Design review of the part built by this model. Coordinates are the model's own, in mm. A direction names the side the tool comes from. Give positions to 0.01 mm unless a question says otherwise; leave off trailing zeros. Write each loop counter-clockwise with the first axis right and the second up, starting at its lowest first coordinate (ties: lowest second). Pieces come first, ordered by that corner, then holes. Notation, with made-up numbers: M 50.5,4 L 70.5,4 A25 cw 70.5,24 Z; hole C 84.5,18.5 d2. An arc over 180 degrees is marked long. Use a Markdown table: item, result. Add a question column.
```python
from build123d import *

# Parameters (mm, degrees)
SKETCH1_W               = 19.05
SKETCH1_H               = 19.05
SKETCH1_W_2             = 15.748
SKETCH1_H_2             = 15.748
BOSS_EXTRUDE1_DEPTH     = 28.575
CUT_EXTRUDE5_DEPTH      = 36.639286609
CUT_EXTRUDE5_DEPTH_BACK = 36.639286609
SKETCH5_R               = 12.7
CUT_EXTRUDE2_DEPTH      = 36.639286609
CUT_EXTRUDE2_DEPTH_BACK = 36.639286609
SKETCH3_R               = 4.064
CUT_EXTRUDE4_DEPTH      = 36.639286609
CUT_EXTRUDE4_DEPTH_BACK = 36.639286609
SKETCH4_W               = 15.748
SKETCH4_H               = 19.05
FILLET2_R               = 6.35


with BuildPart() as part:
    # Sketch1 → Boss-Extrude1 (new body)
    with BuildSketch(Plane.XY):
        Rectangle(SKETCH1_W, SKETCH1_H)
        Rectangle(SKETCH1_W_2, SKETCH1_H_2, mode=Mode.SUBTRACT)
    extrude(amount=BOSS_EXTRUDE1_DEPTH)

    # Sketch5 → Cut-Extrude5 (cut, two sides: drawn at the far end of the back side and taken through both)
    with BuildSketch(Plane(origin=(0, 9.525, 0), x_dir=(1, 0, 0), z_dir=(0, 1, 0)).offset(-CUT_EXTRUDE5_DEPTH_BACK)):
        with Locations((0, 8.400260413)):
            Circle(SKETCH5_R)
    extrude(amount=CUT_EXTRUDE5_DEPTH + CUT_EXTRUDE5_DEPTH_BACK, mode=Mode.SUBTRACT)

    # Sketch3 → Cut-Extrude2 (cut, two sides: drawn at the far end of the back side and taken through both)
    with BuildSketch(Plane(origin=(9.525, 0, 0), x_dir=(0, 0, -1), z_dir=(1, 0, 0)).offset(-CUT_EXTRUDE2_DEPTH_BACK)):
        with Locations(Location((-20.6375, 0, 0), (0, 0, 90))):
            Circle(SKETCH3_R)
    extrude(amount=CUT_EXTRUDE2_DEPTH + CUT_EXTRUDE2_DEPTH_BACK, mode=Mode.SUBTRACT)

    # Sketch4 → Cut-Extrude4 (cut, two sides: drawn at the far end of the back side and taken through both)
    with BuildSketch(Plane.XZ.offset(9.525).offset(-CUT_EXTRUDE4_DEPTH_BACK)):
        with Locations((0, 19.05)):
            Rectangle(SKETCH4_W, SKETCH4_H)
    extrude(amount=CUT_EXTRUDE4_DEPTH + CUT_EXTRUDE4_DEPTH_BACK, mode=Mode.SUBTRACT)

    # Fillet2
    fillet2_edges = [part.edges().sort_by_distance(p)[0] for p in [
        (-8.6995, -9.525, 28.575),
        (8.6995, -9.525, 28.575),
        (-8.6995, 9.525, 28.575),
        (8.6995, 9.525, 28.575),
    ]]
    fillet(fillet2_edges, radius=FILLET2_R)


solid = part.part
```
(1) Wall thickness on L1, parallel to X at y = 0, z = 6 (3 decimals); L2, parallel to Z at x = 8.6, y = 0 (1 decimal): over which ranges is each line inside the solid? List them lowest first.
(2) For pin 1 (1.3 mm diameter, centred on x = 0.5, y = 8.5, fed in from +Z) (3 decimals); pin 2 (5 mm diameter, centred on y = 0, z = 20.64, fed in from +X), all flat-tipped, find the tip position at first contact; note any pin that passes through.
(3) Add section C-C on z = 12.75. Give the boundary of the cut face in (x, y) (3 decimals), then the cut area to 3 significant figures.
(4) The part is to be moulded in two halves that separate along X. For faces 1 (the flat face through (0, -7.874, 6)), 2 (the flat face through (9.525, 0, 14)), 3 (the flat face through (-9.525, 0, 14)), 4 (the cylindrical face through (8.688, 2.185, 24.064)), say which applies: released by +X, released by -X, zero draft, split by the parting line, or undercut.
(5) Add section B-B on y = 0. Give the boundary of the cut face in (x, z) (1 decimal).
(6) Add section A-A on z = 7.25. Give the boundary of the cut face in (x, y) (3 decimals), then the cut area to 3 significant figures.
(7) Machinability: for faces 5 (the flat face through (0, 9, 9.525)), 6 (the cylindrical face through (8.71, -7.62, 26.76)), 7 (the flat face through (-7.874, 0, 15)), 8 (the flat face through (0, 7.874, 6)), which of the approach directions +Z, -Z, +X, -X, +Y, -Y give a long, thin tool a straight path to every point of the face, cutting with its end or side? Answer none if there is none.
(8) Add section D-D on y = 5.25. Give the boundary of the cut face in (x, z) (3 decimals), then the cut area to 3 significant figures.
From the geometry:
| question | item | result |
|---|---|---|
| 1 | L1 | x = -9.525 to -7.874, 7.874 to 9.525 |
| 1 | L2 | z = 0.9 to 16.6, 24.7 to 28.6 |
| 2 | pin 1 | stops at z = 9.525 |
| 2 | pin 2 | passes through |
| 3 | outline | M -9.525,-9.525 L -7.874,-9.525 L -7.874,9.525 L -9.525,9.525 Z; M 7.874,-9.525 L 9.525,-9.525 L 9.525,9.525 L 7.874,9.525 Z |
| 3 | area | 62.9 mm^2 |
| 4 | face 1 | undercut |
| 4 | face 2 | released by +X |
| 4 | face 3 | released by -X |
| 4 | face 4 | zero draft |
| 5 | outline | M -9.5,0 A12.7 cw -7.9,1.6 L -7.9,16.6 L -9.5,16.6 Z; M -9.5,24.7 L -7.9,24.7 L -7.9,28.6 L -9.5,28.6 Z; M 7.9,1.6 A12.7 cw 9.5,0 L 9.5,16.6 L 7.9,16.6 Z; M 7.9,24.7 L 9.5,24.7 L 9.5,28.6 L 7.9,28.6 Z |
| 6 | outline | M -9.525,-9.525 L 9.525,-9.525 L 9.525,9.525 L -9.525,9.525 Z; hole M -7.874,-7.874 L 7.874,-7.874 L 7.874,7.874 L -7.874,7.874 Z |
| 6 | area | 115 mm^2 |
| 7 | face 5 | +Z, +Y, -Y |
| 7 | face 6 | +Z, +X, -X, -Y |
| 7 | face 7 | +Z |
| 7 | face 8 | +Z, -Z |
| 8 | outline | M -9.525,0 A12.7 cw -7.874,1.564 L -7.874,28.226 L -9.525,28.226 Z; M 7.874,1.564 A12.7 cw 9.525,0 L 9.525,28.226 L 7.874,28.226 Z |
| 8 | area | 90.5 mm^2 |
